Geometry: final body of the model. Coordinates: model frame, mm. Round coordinates to 2 decimals unless told otherwise and drop trailing zeros. Loops run counter-clockwise (first coordinate to the right, second up) from the corner with the lowest first, then second, coordinate; pieces in that order, holes last. Notation, with made-up numbers: (-38, 12.5) - (-10, 12.5) arc R19 ccw to (-10, 40.5) - close; hole circle Ø6 at (29, 57.25). An arc over 180 degrees is marked (long way). Write item = value, one per line. Start each with the question number.
Item 1: First-contact query: pin 1 (8 mm diameter, centred on x = -3.5, y = 1.5, fed in from -Z); pin 2 (12 mm diameter, centred on x = 0, y = 0, fed in from -Z). Flat tips, straight axial feed; report the tip coordinate or a pass-through.
Item 2: Section B-B (z = 0.5). Return loops of the section in (x, y).
Item 3: Line query: line 1 (Y direction, x = 6.5, z = 0.75); line 2 (Y direction, x = -5.75, z = 1.5); line 3 (X direction, y = -5, z = 4.25). Output: solid intervals per line, ascending. Write a range as from..to.
Item 4: Section C-C (z = 6). Return loops of the section in (x, y), plus the area to 3 significant figures.
Item 5: Section A-A (z = 4.5). Return loops of the section in (x, y).
from build123d import *

# Parameters (mm, degrees)
SKETCH1_R               = 7.5
BOSS_EXTRUDE1_DEPTH     = 6.58
SKETCH2_OUTSIDE_W       = 43.878
SKETCH2_OUTSIDE_H       = 47.266
SKETCH2_OUTSIDE_R       = 10.95
CUT_EXTRUDE1_DEPTH      = 6.58
CUT_EXTRUDE1_DRAFT      = -45
MIRROR1_COPY_1_SKETCH_W = 43.878
MIRROR1_COPY_1_SKETCH_H = 47.266
MIRROR1_COPY_1_SKETCH_R = 10.95
MIRROR1_COPY_1_DEPTH    = 6.58
MIRROR1_COPY_1_DRAFT    = -45


with BuildPart() as part:
    # Sketch1 → Boss-Extrude1 (new body)
    with BuildSketch(Plane.XY):
        Polygon((0, 12.643970895), (-10.95, 6.321985448), (-10.95, -6.321985448), (0, -12.643970895), (10.95, -6.321985448), (10.95, 6.321985448), align=None)
        with Locations(Location((0, 0, 0), (0, 0, 180))):
            Circle(SKETCH1_R, mode=Mode.SUBTRACT)
    extrude(amount=BOSS_EXTRUDE1_DEPTH)


with BuildPart() as cut_extrude1_tool:
    # Sketch2 outside → Cut-Extrude1 (with draft: the straight prism first)
    with BuildSketch(Plane.XY.offset(6.58)):
        Rectangle(SKETCH2_OUTSIDE_W, SKETCH2_OUTSIDE_H)
        Circle(SKETCH2_OUTSIDE_R, mode=Mode.SUBTRACT)
    extrude(amount=-CUT_EXTRUDE1_DEPTH)
    # Cut-Extrude1: the draft: its side faces are tilted about the plane it starts from
    cut_extrude1_sides = [cut_extrude1_tool.faces().sort_by_distance(p)[0] for p in [
        (0, -23.633, 3.29),
        (21.939, 0, 3.29),
        (0, 23.633, 3.29),
        (-21.939, 0, 3.29),
        (-10.95, 0, 3.29),
    ]]
    draft(cut_extrude1_sides, Plane.XY.offset(6.58), CUT_EXTRUDE1_DRAFT)


with BuildPart() as part_1:
    add(part.part)

    # Cut-Extrude1: cut by cut_extrude1_tool
    add(cut_extrude1_tool.part, mode=Mode.SUBTRACT)


with BuildPart() as mirror1_copy_1_tool:
    # Mirror1 copy 1 sketch → Mirror1 copy 1 (with draft: the straight prism first)
    with BuildSketch(Plane(origin=(0, 0, 0), x_dir=(1, 0, 0), z_dir=(0, 0, -1))):
        Rectangle(MIRROR1_COPY_1_SKETCH_W, MIRROR1_COPY_1_SKETCH_H)
        Circle(MIRROR1_COPY_1_SKETCH_R, mode=Mode.SUBTRACT)
    extrude(amount=-MIRROR1_COPY_1_DEPTH)
    # Mirror1 copy 1: the draft: its side faces are tilted about the plane it starts from
    mirror1_copy_1_sides = [mirror1_copy_1_tool.faces().sort_by_distance(p)[0] for p in [
        (0, -23.633, 3.29),
        (21.939, 0, 3.29),
        (0, 23.633, 3.29),
        (-21.939, 0, 3.29),
        (-10.95, 0, 3.29),
    ]]
    draft(mirror1_copy_1_sides, Plane(origin=(0, 0, 0), x_dir=(1, 0, 0), z_dir=(0, 0, -1)), MIRROR1_COPY_1_DRAFT)


with BuildPart() as part_2:
    add(part_1.part)

    # Mirror1 copy 1: cut by mirror1_copy_1_tool
    add(mirror1_copy_1_tool.part, mode=Mode.SUBTRACT)


solid = part_2.part
Taken from the geometry:
q1.pin_1 = 0
q1.pin_2 = through
q2.outline = (-10.95, -3.35) arc R11.45 ccw to (-8.37, -7.81) - (-2.58, -11.16) arc R11.45 ccw to (2.58, -11.16) - (8.37, -7.81) arc R11.45 ccw to (10.95, -3.35) - (10.95, 3.35) arc R11.45 ccw to (8.37, 7.81) - (2.58, 11.16) arc R11.45 ccw to (-2.58, 11.16) - (-8.37, 7.81) arc R11.45 ccw to (-10.95, 3.35) - close; hole circle Ø15 at (0, 0)
q3.line_1 = -8.89..-3.74, 3.74..8.89
q3.line_2 = -9.32..-4.82, 4.82..9.32
q3.line_3 = -10.95..-5.59, 5.59..10.95
q4.outline = (-10.95, -3.61) arc R11.53 ccw to (-8.6, -7.68) - (-2.35, -11.29) arc R11.53 ccw to (2.35, -11.29) - (8.6, -7.68) arc R11.53 ccw to (10.95, -3.61) - (10.95, 3.61) arc R11.53 ccw to (8.6, 7.68) - (2.35, 11.29) arc R11.53 ccw to (-2.35, 11.29) - (-8.6, 7.68) arc R11.53 ccw to (-10.95, 3.61) - close; hole circle Ø15 at (0, 0)
q4.area = 224 mm^2
q5.outline = (-10.95, -6.32) - (0, -12.64) - (10.95, -6.32) - (10.95, 6.32) - (0, 12.64) - (-10.95, 6.32) - close; hole circle Ø15 at (0, 0)
